The listing builds one solid part. Answer for the finished solid, in the listing's coordinates (mm). A direction names the side the tool comes from. Coordinates: 2 decimals unless noted, no trailing zeros. Loops run counter-clockwise (first coordinate to the right, second up) from the corner with the lowest first, then second, coordinate; pieces in that order, holes last. Notation, with made-up numbers: (31, 49) -> (60, 49) arc R37 ccw to (60, 86) -> close; hole circle Ø6 at (-34, 78.5). An arc over 180 degrees is marked (long way). Answer in a Markdown table with one row per item.
```python
from build123d import *

# Parameters (mm, degrees)
SKETCH1_R           = 1.6
SKETCH1_R_2         = 5.5
BOSS_EXTRUDE1_DEPTH = 3
SKETCH2_R           = 8.025
CUT_EXTRUDE1_DEPTH  = 2


with BuildPart() as part:
    # Sketch1 → Boss-Extrude1 (new body)
    with BuildSketch(Plane(origin=(0, 0, 0), x_dir=(1, 0, 0), z_dir=(0, 1, 0))):
        with BuildLine():
            Line((21.5, -32.43), (-21.5, -32.43))
            ThreePointArc((-21.5, -32.43), (-25.035533906, -30.965533906), (-26.5, -27.43))
            Line((-26.5, -27.43), (-26.5, 8.956951673))
            ThreePointArc((-26.5, 8.956951673), (-25.948126611, 11.731406557), (-24.376524164, 14.083475836))
            Line((-24.376524164, 14.083475836), (-14.728099577, 23.731900423))
            ThreePointArc((-14.728099577, 23.731900423), (-11.263258212, 26.047033407), (-7.176199154, 26.86))
            Line((-7.176199154, 26.86), (7.176199154, 26.86))
            ThreePointArc((7.176199154, 26.86), (11.263258212, 26.047033407), (14.728099577, 23.731900423))
            Line((14.728099577, 23.731900423), (24.376524164, 14.083475836))
            ThreePointArc((24.376524164, 14.083475836), (25.948126611, 11.731406557), (26.5, 8.956951673))
            Line((26.5, 8.956951673), (26.5, -27.43))
            ThreePointArc((26.5, -27.43), (25.035533906, -30.965533906), (21.5, -32.43))
        make_face()
        with Locations((21.920310217, 0)):
            Circle(SKETCH1_R, mode=Mode.SUBTRACT)
        with Locations((-21.920310217, 0)):
            Circle(SKETCH1_R, mode=Mode.SUBTRACT)
        Circle(SKETCH1_R_2, mode=Mode.SUBTRACT)
        with Locations((0, 21.920310217)):
            Circle(SKETCH1_R, mode=Mode.SUBTRACT)
        with BuildLine():
            Line((17.45, -23.81), (17.45, -17))
            ThreePointArc((17.45, -17), (20, -14.45), (22.55, -17))
            Line((22.55, -17), (22.55, -23.81))
            ThreePointArc((22.55, -23.81), (20, -26.36), (17.45, -23.81))
        make_face(mode=Mode.SUBTRACT)
        with BuildLine():
            Line((7.45, -23.81), (7.45, -17))
            ThreePointArc((7.45, -17), (10, -14.45), (12.55, -17))
            Line((12.55, -17), (12.55, -23.81))
            ThreePointArc((12.55, -23.81), (10, -26.36), (7.45, -23.81))
        make_face(mode=Mode.SUBTRACT)
        with BuildLine():
            Line((-2.55, -23.81), (-2.55, -17))
            ThreePointArc((-2.55, -17), (0, -14.45), (2.55, -17))
            Line((2.55, -17), (2.55, -23.81))
            ThreePointArc((2.55, -23.81), (0, -26.36), (-2.55, -23.81))
        make_face(mode=Mode.SUBTRACT)
        with BuildLine():
            Line((-12.55, -23.81), (-12.55, -17))
            ThreePointArc((-12.55, -17), (-10, -14.45), (-7.45, -17))
            Line((-7.45, -17), (-7.45, -23.81))
            ThreePointArc((-7.45, -23.81), (-10, -26.36), (-12.55, -23.81))
        make_face(mode=Mode.SUBTRACT)
        with BuildLine():
            Line((-22.55, -23.81), (-22.55, -17))
            ThreePointArc((-22.55, -17), (-20, -14.45), (-17.45, -17))
            Line((-17.45, -17), (-17.45, -23.81))
            ThreePointArc((-17.45, -23.81), (-20, -26.36), (-22.55, -23.81))
        make_face(mode=Mode.SUBTRACT)
    extrude(amount=BOSS_EXTRUDE1_DEPTH)

    # Sketch2 → Cut-Extrude1 (cut)
    with BuildSketch(Plane(origin=(0, 3, 0), x_dir=(1, 0, 0), z_dir=(0, 1, 0))):
        Circle(SKETCH2_R)
    extrude(amount=-CUT_EXTRUDE1_DEPTH, mode=Mode.SUBTRACT)


solid = part.part
```
Item 1: A cutting plane is placed at A-A, the plane z = 22.5. Determine the outline of the cut face in (x, y), plus the area to 3 significant figures.
Findings below:
| item | result |
|---|---|
| outline | (-26.5, 0) -> (-22.55, 0) -> (-22.55, 3) -> (-26.5, 3) -> close; (-17.45, 0) -> (-12.55, 0) -> (-12.55, 3) -> (-17.45, 3) -> close; (-7.45, 0) -> (-2.55, 0) -> (-2.55, 3) -> (-7.45, 3) -> close; (2.55, 0) -> (7.45, 0) -> (7.45, 3) -> (2.55, 3) -> close; (12.55, 0) -> (17.45, 0) -> (17.45, 3) -> (12.55, 3) -> close; (22.55, 0) -> (26.5, 0) -> (26.5, 3) -> (22.55, 3) -> close |
| area | 82.5 mm2 |
Item 2: Flat-ended cylindrical pins translate along their axes: pin 1 Ø6.5 at (x, z) = (0, 0) entering from -Y; pin 2 Ø8 at (x, z) = (-2.5, 0) entering from +Y. Find the tip coordinate at first contact, or state that the pin passes through.
Findings below:
| item | result |
|---|---|
| pin 1 | passes through |
| pin 2 | stops at y = 1 |
Item 3: A cutting plane is placed at D-D, the plane z = -19.5. Determine the outline of the cut face in (x, y), plus the area to 3 significant figures.
Findings below:
| item | result |
|---|---|
| outline | (-18.96, 0) -> (18.96, 0) -> (18.96, 3) -> (-18.96, 3) -> close |
| area | 114 mm2 |
Item 4: A tool of negligible diameter and unlimited length cuts with its end or side. For faces 5 (the face through (25.93, 1.48, -11.77)), 6 (the face through (-6.37, 2.01, 4.88)), 7 (the face through (10.06, 1.48, 26.36)), from which of +Z, -Z, +X, -X, +Y, -Y can it reach the whole face along a straight path? Write none if from no direction.
Findings below:
| item | result |
|---|---|
| face 5 | -Z, +X, +Y, -Y |
| face 6 | +Y |
| face 7 | +Y, -Y |
Item 5: Determine the mould class of faces 1 (the face through (-7.45, 1, 20)), 2 (the face through (17.45, 1, 20)), 3 (the face through (26.5, 1, 9)), 4 (the face through (0, 1, -26.86)) for opening direction Z: +Z half, -Z half, draft (parallel to the pull), parting line (faces both ways), or undercut.
Findings below:
| item | result |
|---|---|
| face 1 | undercut |
| face 2 | undercut |
| face 3 | draft |
| face 4 | -Z half |
Item 6: Find the intervals of material crossed by probe 1 along Z at (x, y) = (0, 0.3); probe 2 along X at (y, z) = (0.8, 0); probe 3 along X at (y, z) = (1.1, 0) (3 decimals), in increasing order.
Findings below:
| item | result |
|---|---|
| probe 1 | z = -26.86 to -23.52, -20.32 to -5.5, 5.5 to 14.45, 26.36 to 32.43 |
| probe 2 | x = -26.5 to -23.52, -20.32 to -5.5, 5.5 to 20.32, 23.52 to 26.5 |
| probe 3 | x = -26.5 to -23.52, -20.32 to -8.025, 8.025 to 20.32, 23.52 to 26.5 |
Item 7: A cutting plane is placed at B-B, the plane z = 0. Determine the outline of the cut face in (x, y) (3 decimals).
Findings below:
| item | result |
|---|---|
| outline | (-26.5, 0) -> (-23.52, 0) -> (-23.52, 3) -> (-26.5, 3) -> close; (-20.32, 0) -> (-5.5, 0) -> (-5.5, 1) -> (-8.025, 1) -> (-8.025, 3) -> (-20.32, 3) -> close; (5.5, 0) -> (20.32, 0) -> (20.32, 3) -> (8.025, 3) -> (8.025, 1) -> (5.5, 1) -> close; (23.52, 0) -> (26.5, 0) -> (26.5, 3) -> (23.52, 3) -> close |
Item 8: A cutting plane is placed at C-C, the plane x = -10. Determine the outline of the cut face in (y, z).
Findings below:
| item | result |
|---|---|
| outline | (0, -26.48) -> (3, -26.48) -> (3, 14.45) -> (0, 14.45) -> close; (0, 26.36) -> (3, 26.36) -> (3, 32.43) -> (0, 32.43) -> close |
